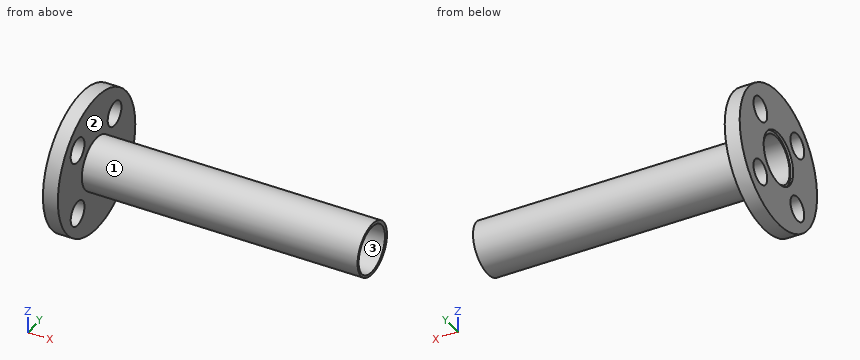
```python
from build123d import *

# Parameters (mm, degrees)
SKETCH3_R          = 15.18
CUT_EXTRUDE1_DEPTH = 187.086523502
SKETCH5_R          = 7.9375
CUT_EXTRUDE2_DEPTH = 10


with BuildPart() as part:
    # Sketch1 → Revolve1 (revolve)
    with BuildSketch(Plane.XY):
        Polygon((53.975, 0.555053367), (53.975, 11.176), (53.975, 17.526), (52.451, 17.526), (52.451, 45.185378607), (62.101, 45.185378607), (62.101, 17.526), (240.061523502, 17.526), (240.061523502, 0.555053367), align=None)
    revolve(axis=Axis((53.975, 0.555053367, 0), (1, 0, 0)))

    # Sketch3 → Cut-Extrude1 (cut, through all)
    with BuildSketch(Plane.ZY.offset(-53.975)):
        Circle(SKETCH3_R)
    extrude(amount=-CUT_EXTRUDE1_DEPTH, mode=Mode.SUBTRACT)

    # Sketch5 → Cut-Extrude2 (cut)
    with BuildSketch(Plane.ZY.offset(-52.451)):
        with Locations((-21.49441643, 21.314234902)):
            Circle(SKETCH5_R)
        with Locations((-21.49441643, -21.341981673)):
            Circle(SKETCH5_R)
        with Locations((21.161800145, 21.314234902)):
            Circle(SKETCH5_R)
        with Locations((21.161800145, -21.341981673)):
            Circle(SKETCH5_R)
    extrude(amount=-CUT_EXTRUDE2_DEPTH, mode=Mode.SUBTRACT)


solid = part.part
```
The model under review builds one solid part; all positions refer to its coordinate system, in mm. Face numbers are marked on the shaded views. Give positions to 0.01 mm unless a question says otherwise; leave off trailing zeros. Write each loop counter-clockwise with the first axis right and the second up, starting at its lowest first coordinate (ties: lowest second). Pieces come first, ordered by that corner, then holes.
(1) Consider section C-C, the plane y = 26. Give the boundary of the cut face in (x, z).
(2) For P1, Ø10, axis at x = 209.5, y = -1, coming from the +Z side; P2, Ø20.5, axis at y = -21.34, z = -21.49, coming from the -X side; P3, Ø6, axis at y = -11.5, z = -19.5, coming from the +X side, all flat-tipped, find the tip position at first contact; note any pin that passes through.
(3) Consider section B-B, the plane y = 0. Give the boundary of the cut face in (x, z) (3 decimals).
(4) Consider section A-A, the plane z = 0. Give the boundary of the cut face in (x, y) (3 decimals).
(5) The part is to be moulded in two halves that separate along Z. For the marked faces 1, 2 and 3, say which applies: released by +Z, released by -Z, zero draft, split by the parting line, or undercut.
(6) Consider section D-D, the plane x = 219.5. Give the boundary of the cut face in (y, z).
(7) To check wall thickness, follow L1, parallel to X at y = 12, z = -41; L2, parallel to X at y = 16, z = -5 (3 decimals); L3, parallel to Y at x = 179, z = 6.5. State the ranges of each line that lie inside material, in increasing order.
Returned:
1. outline: (52.45, -36.67) - (62.1, -36.67) - (62.1, -27.9) - (52.45, -27.9) - close; (52.45, -15.09) - (62.1, -15.09) - (62.1, 14.75) - (52.45, 14.75) - close; (52.45, 27.57) - (62.1, 27.57) - (62.1, 36.67) - (52.45, 36.67) - close
2. P1: stops at z = 16.97
2. P2: stops at x = 52.45
2. P3: stops at x = 62.1
3. outline: (52.451, -44.627) - (62.101, -44.627) - (62.101, -16.962) - (240.062, -16.962) - (240.062, -15.18) - (53.975, -15.18) - (53.975, -16.962) - (52.451, -16.962) - close; (52.451, 16.962) - (53.975, 16.962) - (53.975, 15.18) - (240.062, 15.18) - (240.062, 16.962) - (62.101, 16.962) - (62.101, 44.627) - (52.451, 44.627) - close
4. outline: (52.451, -44.075) - (62.101, -44.075) - (62.101, -16.416) - (240.062, -16.416) - (240.062, -15.18) - (53.975, -15.18) - (53.975, -16.416) - (52.451, -16.416) - close; (52.451, 17.526) - (53.975, 17.526) - (53.975, 15.18) - (240.062, 15.18) - (240.062, 17.526) - (62.101, 17.526) - (62.101, 45.185) - (52.451, 45.185) - close
5. face 1: split by the parting line
5. face 2: zero draft
5. face 3: undercut
6. outline: circle Ø33.94 at (0.56, 0); hole circle Ø30.36 at (0, 0)
7. L1: x = 52.45 to 62.1
7. L2: x = 53.975 to 240.062
7. L3: y = -15.12 to -13.72, 13.72 to 16.23
